from build123d import *

# Parameters (mm, degrees)
PAD144_DEPTH            = 36.3
PAD145_DEPTH            = 36.3
POCKET111_DEPTH         = 28.2
PAD146_DEPTH            = 8.1
POCKET112_DEPTH         = 5.1
POCKET113_DEPTH         = 5.1
POCKET114_DEPTH         = 2
POCKET115_DEPTH         = 22
SKETCH252_W             = 3.1
SKETCH252_H             = 1.9
SKETCH252_H_2           = 2
POCKET116_DEPTH         = 1.7
PAD147_DEPTH            = 36.3
POCKET117_DEPTH         = 34
PAD148_DEPTH            = 2.3
FILLET047_R             = 0.5
BODY021_ROLL_ANGLE      = 90
BODY021_PLACEMENT_ANGLE = 90


with BuildPart() as part:
    # Sketch248 → Pad144 (new body)
    with BuildSketch(Plane.XY):
        Polygon((0, 0), (0, 1.4), (13.5, 1.4), (13.5, 21.4), (15.2, 21.4), (15.2, 0), align=None)
    extrude(amount=PAD144_DEPTH)

    # Sketch249 (on Face8 of Pad144) → Pad145 (join)
    with BuildSketch(Plane.XY.offset(36.3)):
        with BuildLine():
            Line((15.2, 15.6), (20.036303, 14.331076))
            ThreePointArc((20.036303, 8.568924), (22.2, 11.45), (20.036303, 14.331076))
            Line((15.2, 7.3), (20.036303, 8.568924))
            Line((15.2, 7.3), (15.2, 15.6))
        make_face()
    extrude(amount=-PAD145_DEPTH)

    # Sketch249 (on Face8 of Pad144) → Pocket111 (cut)
    with BuildSketch(Plane.XY.offset(36.3)):
        with BuildLine():
            Line((15.2, 15.6), (20.036303, 14.331076))
            ThreePointArc((20.036303, 8.568924), (22.2, 11.45), (20.036303, 14.331076))
            Line((15.2, 7.3), (20.036303, 8.568924))
            Line((15.2, 7.3), (15.2, 15.6))
        make_face()
    extrude(amount=-POCKET111_DEPTH, mode=Mode.SUBTRACT)

    # Sketch249 (on Face8 of Pad144) → Pad146 (join)
    with BuildSketch(Plane.XY.offset(36.3)):
        with BuildLine():
            Line((15.2, 15.6), (20.036303, 14.331076))
            ThreePointArc((20.036303, 8.568924), (22.2, 11.45), (20.036303, 14.331076))
            Line((15.2, 7.3), (20.036303, 8.568924))
            Line((15.2, 7.3), (15.2, 15.6))
        make_face()
    extrude(amount=-PAD146_DEPTH)

    # Sketch249 (on Face8 of Pad144) → Pocket112 (cut)
    with BuildSketch(Plane.XY.offset(36.3)):
        with BuildLine():
            Line((15.2, 15.6), (20.036303, 14.331076))
            ThreePointArc((20.036303, 8.568924), (22.2, 11.45), (20.036303, 14.331076))
            Line((15.2, 7.3), (20.036303, 8.568924))
            Line((15.2, 7.3), (15.2, 15.6))
        make_face()
    extrude(amount=-POCKET112_DEPTH, mode=Mode.SUBTRACT)

    # Sketch250 (on Face4 of Pocket112) → Pocket113 (cut)
    with BuildSketch(Plane(origin=(0, 0, 0), x_dir=(1, 0, 0), z_dir=(0, 0, -1))):
        with BuildLine():
            Line((20.036303, -8.568924), (15.2, -7.3))
            Line((15.2, -7.3), (15.2, -15.6))
            Line((15.2, -15.6), (20.036303, -14.331076))
            ThreePointArc((20.036303, -14.331076), (22.2, -11.45), (20.036303, -8.568924))
        make_face()
    extrude(amount=-POCKET113_DEPTH, mode=Mode.SUBTRACT)

    # Sketch251 (on Face15 of Pocket113) → Pocket114 (cut)
    with BuildSketch(Plane.XY.offset(8.1)):
        with BuildLine():
            ThreePointArc((19.2, 9.9), (20.75, 11.45), (19.2, 13))
            Line((19.2, 13), (15.2, 13))
            Line((15.2, 9.9), (15.2, 13))
            Line((19.2, 9.9), (15.2, 9.9))
        make_face()
    extrude(amount=-POCKET114_DEPTH, mode=Mode.SUBTRACT)

    # Sketch251 (on Face15 of Pocket113) → Pocket115 (cut)
    with BuildSketch(Plane.XY.offset(8.1)):
        with BuildLine():
            ThreePointArc((19.2, 9.9), (20.75, 11.45), (19.2, 13))
            Line((19.2, 13), (15.2, 13))
            Line((15.2, 9.9), (15.2, 13))
            Line((19.2, 9.9), (15.2, 9.9))
        make_face()
    extrude(amount=POCKET115_DEPTH, mode=Mode.SUBTRACT)

    # Sketch252 (on Face8 of Pocket115) → Pocket116 (cut)
    with BuildSketch(Plane.YZ.offset(15.2)):
        with Locations((11.45, 29.15)):
            Rectangle(SKETCH252_W, SKETCH252_H)
        with Locations((11.45, 7.1)):
            Rectangle(SKETCH252_W, SKETCH252_H_2)
    extrude(amount=-POCKET116_DEPTH, mode=Mode.SUBTRACT)

    # Sketch253 (on Face5 of Pocket116) → Pad147 (join)
    with BuildSketch(Plane.XY.offset(36.3)):
        with BuildLine():
            Line((13.5, 21.4), (13.5, 1.4))
            Line((13.5, 1.4), (2, 1.4))
            ThreePointArc((2, 1.4), (2.384708, 1.498573), (2.674611, 1.77))
            Line((2.674611, 1.77), (13.5, 21.4))
        make_face()
    extrude(amount=-PAD147_DEPTH)

    # Sketch253 (on Face5 of Pocket116) → Pocket117 (cut)
    with BuildSketch(Plane.XY.offset(36.3)):
        with BuildLine():
            Line((13.5, 21.4), (13.5, 1.4))
            Line((13.5, 1.4), (2, 1.4))
            ThreePointArc((2, 1.4), (2.384708, 1.498573), (2.674611, 1.77))
            Line((2.674611, 1.77), (13.5, 21.4))
        make_face()
    extrude(amount=-POCKET117_DEPTH, mode=Mode.SUBTRACT)

    # Sketch253 (on Face5 of Pocket116) → Pad148 (join)
    with BuildSketch(Plane.XY.offset(36.3)):
        with BuildLine():
            Line((13.5, 21.4), (13.5, 1.4))
            Line((13.5, 1.4), (2, 1.4))
            ThreePointArc((2, 1.4), (2.384708, 1.498573), (2.674611, 1.77))
            Line((2.674611, 1.77), (13.5, 21.4))
        make_face()
    extrude(amount=-PAD148_DEPTH)

    # Fillet047
    fillet047_edges = [part.edges().sort_by_distance(p)[0] for p in [
        (7.6, 0, 36.3),
        (15.2, 10.7, 36.3),
        (15.2, 0, 18.15),
        (15.2, 10.7, 0),
        (7.6, 0, 0),
    ]]
    fillet(fillet047_edges, radius=FILLET047_R)


with BuildPart() as part_1:
    # Body021 roll: moved
    add(part.part.rotate(Axis((0, 0, 0), (1, 0, 0)), BODY021_ROLL_ANGLE))


with BuildPart() as part_2:
    # Body021 placement: moved
    add(part_1.part.moved(Location((20.05, -79.35, -11.45))).rotate(Axis((20.05, -79.35, -11.45), (0, 0, 1)), BODY021_PLACEMENT_ANGLE))


solid = part_2.part
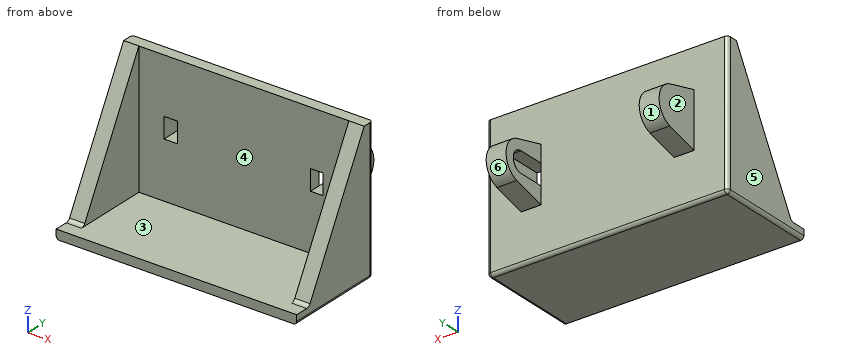
Can you work these out from the model? Positions are in its coordinate system, mm. Face numbers are marked on the shaded views. A direction names the side the tool comes from. Round coordinates to 2 decimals unless told otherwise and drop trailing zeros. Loops run counter-clockwise (first coordinate to the right, second up) from the corner with the lowest first, then second, coordinate; pieces in that order, holes last. Notation, with made-up numbers: (42, 63) - (59, 63) arc R13 cw to (59, 79) - close; hole circle Ø7 at (-6, 21.5). An arc over 180 degrees is marked (long way). Write item = value, one per line. Start each with the question number.
(1) For the marked faces 1, 2 and 3, which set-ups out of +Z, -Z, +X, -X, +Y, -Y let a thin tool reach every point of the face, with its end or its side?
(2) For P1, Ø1, axis at x = 27, y = -63, coming from the +Z side; P2, Ø5, axis at x = 49.5, z = 4, coming from the +Y side; P3, Ø2, axis at x = 39.5, z = 3.5, coming from the +Y side, each with a flat end and sliding along its axis, tell me the tip position at first contact or that it passes through.
(3) If we mould it in two halves opening along X, with no side actions, what happens to the marked faces 4, 5 and 6? For each: released by +X, released by -X, zero draft, split by the parting line, or undercut.
(4) If we section it at B-B (y = -69.5): Please give me the cut outline in (x, z), and give its area (3 significant figures).
(5) If we section it at C-C (z = 5.5): Please give me the cut outline in (x, y), and give its area (3 significant figures).
(6) If I drill on probe 1 along X at (y, z) = (-65.75, -0.25); probe 2 along X at (y, z) = (-70.5, -3.5); probe 3 along X at (y, z) = (-63.5, -1.25), over which ranges is the centre line in solid material (lowest first)? Write a range as [from, to].
(7) If we section it at A-A (z = 0): Please give me the cut outline in (x, y).
Ans:
q1.face_1 = +X, -X, +Y
q1.face_2 = +Z, -Z, -X, +Y
q1.face_3 = +Z, -Y
q2.P1 = 3.98
q2.P2 = -57.55
q2.P3 = -64.15
q3.face_4 = undercut
q3.face_5 = released by -X
q3.face_6 = zero draft
q4.outline = (20.05, -10.95) arc R0.5 ccw to (20.55, -11.45) - (55.85, -11.45) arc R0.5 ccw to (56.35, -10.95) - (56.35, 3.33) - (54.05, 3.33) - (54.05, -10.05) - (22.35, -10.05) - (22.35, 3.33) - (20.05, 3.33) - close
q4.area = 112 mm²
q5.outline = (20.05, -68.3) - (22.35, -68.3) - (22.35, -65.85) - (54.05, -65.85) - (54.05, -68.3) - (56.35, -68.3) - (56.35, -64.65) arc R0.5 ccw to (55.85, -64.15) - (20.55, -64.15) arc R0.5 ccw to (20.05, -64.65) - close
q5.area = 72.9 mm²
q6.probe_1 = [20.05, 26.15], [28.15, 48.25], [50.15, 56.35]
q6.probe_2 = [20.05, 22.35], [54.05, 56.35]
q6.probe_3 = [25.15, 26.15], [50.15, 51.25]
q7.outline = (20.05, -71.34) - (22.35, -71.34) - (22.35, -65.85) - (26.15, -65.85) - (26.15, -58.6) - (28.15, -58.6) - (28.15, -57.15) - (25.15, -57.15) - (25.15, -64.15) - (20.55, -64.15) arc R0.5 ccw to (20.05, -64.65) - close; (28.15, -65.85) - (48.25, -65.85) - (48.25, -64.15) - (28.15, -64.15) - close; (48.25, -58.6) - (50.15, -58.6) - (50.15, -65.85) - (54.05, -65.85) - (54.05, -71.34) - (56.35, -71.34) - (56.35, -64.65) arc R0.5 ccw to (55.85, -64.15) - (51.25, -64.15) - (51.25, -57.15) - (48.25, -57.15) - close
